Here's how the part is built. I have some questions about the finished solid (model axes, mm). Face numbers are marked on the shaded views. A direction names the side the tool comes from. Give positions to 0.01 mm unless a question says otherwise; leave off trailing zeros. Loops run counter-clockwise (first coordinate to the right, second up) from the corner with the lowest first, then second, coordinate; pieces in that order, holes last.
Q1. We'd pull the mould along Z, two halves only. Please class the marked faces 1, 2 and 3: +Z half, -Z half, draft (parallel to the pull), parting line (faces both ways), or undercut.
Q2. If we section it at C-C (y = 14.25): Please give me the cut outline in (x, z), plus the area to 3 significant figures.
Q3. I need wall thicknesses on line 1 (Z direction, x = -1.65, y = 7.5); line 2 (X direction, y = 1.1, z = 7.5); line 3 (X direction, y = 13, z = 7.5). Which ranges of each line are inside material? Lowest first, please.
Q4. If we section it at B-B (z = 7): Please give me the cut outline in (x, y).
Q5. If we section it at D-D (y = 7): Please give me the cut outline in (x, z).
Q6. If we section it at A-A (x = -11.75): Please give me the cut outline in (y, z).
Q7. Will these pins go through, and if not, where does the flat tip stop? P1, Ø3, axis at y = 6.5, z = 8.5, coming from the +X side; P2, Ø3, axis at x = -7.5, y = 7.5, coming from the +Z side; P3, Ø5.5, axis at x = -7.5, y = 7.5, coming from the -Z side.
Q8. For the marked faces 4 and 5, which set-ups out of +Z, -Z, +X, -X, +Y, -Y let a thin tool reach every point of the face, with its end or its side?
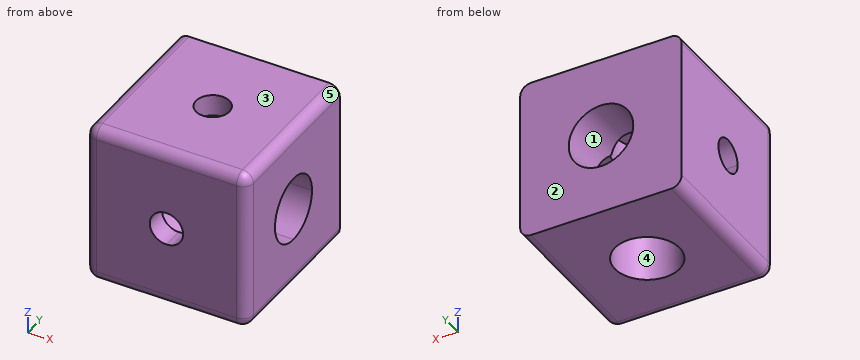
from build123d import *
from build123d import SkipClean  # not in build123d's __all__

# Parameters (mm, degrees)
F0_W      = 15
F0_H      = 15
F1_DEPTH  = 15
F3_DEPTH  = 25
F5_DEPTH  = 25
F7_DEPTH  = 13
F9_DEPTH  = 25
F10_R     = 3
F11_DEPTH = 13
F12_R     = 3
F13_DEPTH = 13
F14_R     = 1


with BuildPart() as f1:
    # F0 (on Top) → F1 (new body)
    with BuildSketch(Plane.XY):
        with Locations((-7.5, 7.5)):
            Rectangle(F0_W, F0_H)
    extrude(amount=F1_DEPTH)

    # F2 (on face) → F3 (cut)
    with BuildSketch(Plane.XZ):
        with BuildLine():
            ThreePointArc((-7.5, 5.95), (-6.4039844892, 6.4039844892), (-5.95, 7.5))
            ThreePointArc((-5.95, 7.5), (-8.5960155108, 8.5960155108), (-7.5, 5.95))
        make_face()
    extrude(amount=-F3_DEPTH, mode=Mode.SUBTRACT)

    # F4 (on face) → F5 (cut)
    with BuildSketch(Plane.XY.offset(15)):
        with BuildLine():
            ThreePointArc((-7.5, 5.95), (-6.4039844892, 6.4039844892), (-5.95, 7.5))
            ThreePointArc((-5.95, 7.5), (-8.5960155108, 8.5960155108), (-7.5, 5.95))
        make_face()
    extrude(amount=-F5_DEPTH, mode=Mode.SUBTRACT)

    # F6 (on face) → F7 (cut)
    with BuildSketch(Plane.YZ):
        with BuildLine():
            ThreePointArc((7.5, 4.5), (9.6213203436, 5.3786796564), (10.5, 7.5))
            ThreePointArc((10.5, 7.5), (5.3786796564, 9.6213203436), (7.5, 4.5))
        make_face()
    with SkipClean():  # cleaning this boolean's faces spoils the solid; the shape is the same uncleaned
        extrude(amount=-F7_DEPTH, mode=Mode.SUBTRACT)

    # F8 (on face) → F9 (cut)
    with BuildSketch(Plane(origin=(-15, 0, 0), x_dir=(0, -1, 0), z_dir=(-1, 0, 0))):
        with BuildLine():
            ThreePointArc((-7.5, 5.95), (-6.4039844892, 6.4039844892), (-5.95, 7.5))
            ThreePointArc((-5.95, 7.5), (-8.5960155108, 8.5960155108), (-7.5, 5.95))
        make_face()
    with SkipClean():  # cleaning this boolean's faces spoils the solid; the shape is the same uncleaned
        extrude(amount=-F9_DEPTH, mode=Mode.SUBTRACT)

    # F10 (on face) → F11 (cut)
    with BuildSketch(Plane(origin=(0, 15, 0), x_dir=(-1, 0, 0), z_dir=(0, 1, 0))):
        with Locations((7.5, 7.5)):
            Circle(F10_R)
    extrude(amount=-F11_DEPTH, mode=Mode.SUBTRACT)

    # F12 (on face) → F13 (cut)
    with BuildSketch(Plane(origin=(0, 0, 0), x_dir=(1, 0, 0), z_dir=(0, 0, -1))):
        with Locations((-7.5, -7.5)):
            Circle(F12_R)
    extrude(amount=-F13_DEPTH, mode=Mode.SUBTRACT)

    # F14
    f14_edges = [f1.edges().sort_by_distance(p)[0] for p in [
        (-15, 0, 7.5),
        (-7.5, 0, 0),
        (0, 0, 7.5),
        (-7.5, 0, 15),
        (-15, 7.5, 0),
        (-15, 7.5, 15),
        (0, 7.5, 15),
        (0, 7.5, 0),
    ]]
    fillet(f14_edges, radius=F14_R)


solid = f1.part
Check sheet entries:
1. face 1: undercut
1. face 2: draft
1. face 3: +Z half
2. outline: (-15, 1) arc R1 ccw to (-14, 0) - (-1, 0) arc R1 ccw to (0, 1) - (0, 14) arc R1 ccw to (-1, 15) - (-14, 15) arc R1 ccw to (-15, 14) - close; hole circle Ø6 at (-7.5, 7.5)
2. area: 196 mm2
3. line 1: z = 0 to 4.5, 10.5 to 15
3. line 2: x = -15 to -9.05, -5.95 to 0
3. line 3: x = -15 to -10.5, -4.5 to 0
4. outline: (-15, 1) arc R1 ccw to (-14, 0) - (-8.97, 0) - (-8.97, 2) - (-10.46, 2) - (-10.46, 4.54) - (-13, 4.54) - (-13, 6.03) - (-15, 6.03) - close; (-15, 8.97) - (-13, 8.97) - (-13, 10.46) - (-10.46, 10.46) - (-10.46, 15) - (-15, 15) - close; (-6.03, 0) - (-1, 0) arc R1 ccw to (0, 1) - (0, 4.54) - (-4.54, 4.54) - (-4.54, 2) - (-6.03, 2) - close; (-4.54, 10.46) - (0, 10.46) - (0, 15) - (-4.54, 15) - close
5. outline: (-15, 1) arc R1 ccw to (-14, 0) - (-10.46, 0) - (-10.46, 4.54) - (-13, 4.54) - (-13, 6.03) - (-15, 6.03) - close; (-15, 8.97) - (-13, 8.97) - (-13, 10.46) - (-10.46, 10.46) - (-10.46, 13) - (-8.97, 13) - (-8.97, 15) - (-14, 15) arc R1 ccw to (-15, 14) - close; (-6.03, 13) - (-4.54, 13) - (-4.54, 10.46) - (0, 10.46) - (0, 14) arc R1 ccw to (-1, 15) - (-6.03, 15) - close; (-4.54, 0) - (-1, 0) arc R1 ccw to (0, 1) - (0, 4.54) - (-4.54, 4.54) - close
6. outline: (0, 1) arc R1 ccw to (1, 0) - (15, 0) - (15, 15) - (1, 15) arc R1 ccw to (0, 14) - close; hole circle Ø6 at (7.5, 7.5)
7. P1: stops at x = -13
7. P2: passes through
7. P3: stops at z = 13
8. face 4: -Z
8. face 5: +Z, +X, +Y, -Y
